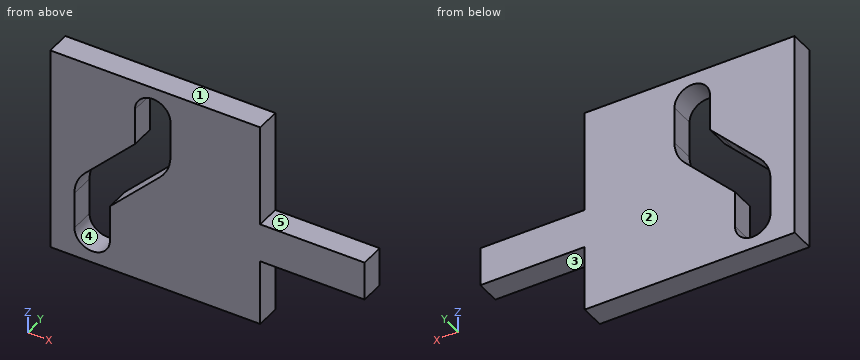
from build123d import *

# Parameters (mm, degrees)
F1_DEPTH = 8.89


# Not quite as in the source:
# - ends of sketch curves that miss each other by under 0.0002 mm in the source are joined


with BuildPart() as f1:
    # F0 (on Front) → F1 (new body)
    with BuildSketch(Plane.XZ):
        Polygon((49.2809079587, 38.859821856), (0, 38.859821856), (-27.3745507002, 38.859821856), (-27.3745507002, 1.9207646612), (-27.3745507002, -36.7616191506), (49.2809079587, -36.7616191506), (49.2809079587, -12.6536535591), (87.395709982, -12.6536535591), (87.395709982, -5.5416535591), (87.395709982, 1.5703464409), (49.2809079587, 1.5703464409), align=None)
        with BuildLine():
            Line((-5.6126600757, 5.6126600757), (0, 11.2253201513))
            Line((0, 11.2253201513), (3.5468912197, 14.7722113711))
            Line((3.5468912197, 14.7722113711), (3.5468912197, 28.1402313711))
            ThreePointArc((3.5468912197, 28.1402313711), (10.0238912197, 34.6172313711), (16.5008912197, 28.1402313711))
            Line((16.5008912197, 28.1402313711), (16.5008912197, 14.7722113711))
            ThreePointArc((16.5008912197, 14.7722113711), (15.5148266839, 9.8149301882), (12.7067524632, 5.6123501276))
            Line((12.7067524632, 5.6123501276), (3.5517127264, -3.5426896092))
            Line((3.5517127264, -3.5426896092), (-5.6081485171, -12.7025508527))
            Line((-5.6081485171, -12.7025508527), (-5.6081485171, -26.002401486))
            ThreePointArc((-5.6081485171, -26.002401486), (-12.085148378, -32.479401347), (-18.562148239, -26.002401486))
            Line((-18.562148239, -26.002401486), (-18.562148239, -12.7025505746))
            ThreePointArc((-18.562148239, -12.7025505746), (-17.5773042343, -7.7482170412), (-14.7725202074, -3.5472022785))
            Line((-14.7725202074, -3.5472022785), (-14.7680094825, -3.5426893311))
            Line((-14.7680094825, -3.5426893311), (-5.6129700238, 5.6123501276))
            Line((-5.6129700238, 5.6123501276), (-5.6126600757, 5.6126600757))
        make_face(mode=Mode.SUBTRACT)
    extrude(amount=F1_DEPTH)


solid = f1.part
Can you work these out from the model? Positions are in its coordinate system, mm. Face numbers are marked on the shaded views. A direction names the side the tool comes from. Round coordinates to 2 decimals unless told otherwise and drop trailing zeros. Write each loop counter-clockwise with the first axis right and the second up, starting at its lowest first coordinate (ties: lowest second). Pieces come first, ordered by that corner, then holes. Notation, with made-up numbers: (48.25, 66.25) - (70.25, 66.25) arc R8 ccw to (70.25, 71.25) - close; hole circle Ø2 at (63.5, -4.5). An arc over 180 degrees is marked (long way). Write each question's results on one line, items separated by ' | '. Start each with the question number.
1) For pin 1 Ø2 at (y, z) = (-5, 18.5) entering from +X; pin 2 Ø5 at (x, y) = (74.5, -7) entering from +Z; pin 3 Ø4.5 at (x, y) = (61, -6) entering from -Z, each with a flat end and sliding along its axis, tell me the tip position at first contact or that it passes through.
2) Which directions (+Z, -Z, +X, -X, +Y, -Y) give clear straight access to the entire face, cutting with the end or side of a thin tool? Please do the marked faces 1, 2, 3, 4 and 5.
3) Suppose I cut it at D-D (z = -8). List the corners of the cut face in (x, y) for me, and give its area (3 significant figures).
4) Please list where these lines run through material, in increasing order: line 1 (X direction, y = -4.5, z = -1.5); line 2 (X direction, y = -3.25, z = -18.5); line 3 (Z direction, x = 74.5, y = -5).
5) Suppose I cut it at C-C (x = 71). List the corners of the cut face in (y, z) for me, and give its area (3 significant figures).
6) Suppose I cut it at A-A (z = -23). List the corners of the cut face in (x, y) for me.
Here are the results:
1) pin 1: stops at x = 49.28 | pin 2: stops at z = 1.57 | pin 3: stops at z = -12.65
2) face 1: +Z, +X, -X, +Y, -Y | face 2: +Z, -Z, +X, -X, +Y | face 3: -Z, +X, +Y, -Y | face 4: +Y, -Y | face 5: +Z, +X, +Y, -Y
3) outline: (-27.37, -8.89) - (-17.68, -8.89) - (-17.68, 0) - (-27.37, 0) - close; (-0.91, -8.89) - (87.4, -8.89) - (87.4, 0) - (-0.91, 0) - close | area: 871 mm2
4) line 1: x = -27.37 to -12.73, 5.59 to 87.4 | line 2: x = -27.37 to -18.56, -5.61 to 49.28 | line 3: z = -12.65 to 1.57
5) outline: (-8.89, -12.65) - (0, -12.65) - (0, 1.57) - (-8.89, 1.57) - close | area: 126 mm2
6) outline: (-27.37, -8.89) - (-18.56, -8.89) - (-18.56, 0) - (-27.37, 0) - close; (-5.61, -8.89) - (49.28, -8.89) - (49.28, 0) - (-5.61, 0) - close
